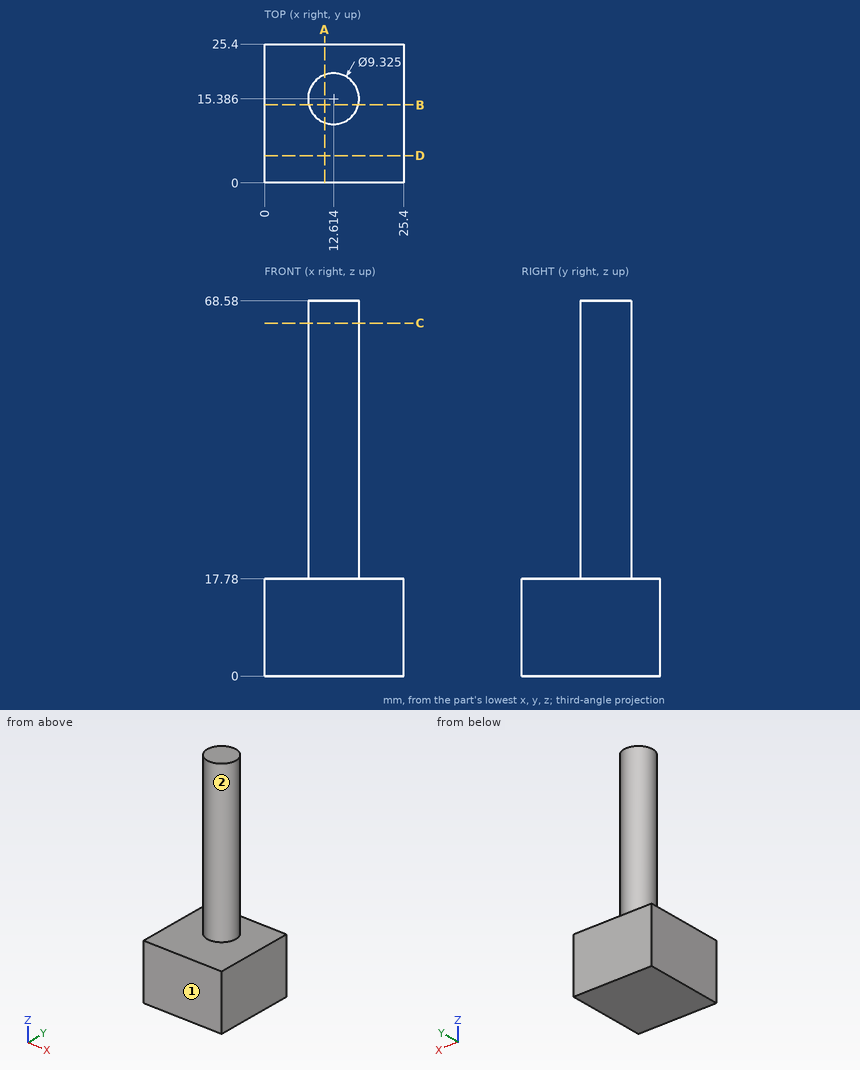
Can you work these out from the drawing? Everything is in mm from the part's minimum corner. A direction names the side the tool comes from. Round coordinates to 2 decimals unless told otherwise and drop trailing zeros. Write each loop counter-clockwise with the first axis right and the second up, starting at its lowest first coordinate (ties: lowest second). Pieces come first, ordered by that corner, then holes. Notation, with made-up numbers: (62, 43.25) - (110, 43.25) arc R24 ccw to (110, 65.25) - close; hole circle Ø3 at (-35.5, 56). An arc over 180 degrees is marked (long way). Write each question's results on one line, items separated by ' | '. Start each with the question number.
1) Suppose I cut it at A-A (x = 11). List the corners of the cut face in (y, z) for me.
2) Suppose I cut it at D-D (y = 5). List the corners of the cut face in (x, z) for me.
3) For pin 1 Ø3 at (y, z) = (19, 19.5) entering from +X; pin 2 Ø4 at (y, z) = (10, 25) entering from -X; pin 3 Ø3 at (y, z) = (16, 61) entering from -X, each with a flat end and sliding along its axis, tell me the tip position at first contact or that it passes through.
4) Suppose I cut it at C-C (z = 64.5). List the corners of the cut face in (x, y) for me (1 decimal).
5) Please list where these lines run through material, in increasing order: line 1 (Z direction, x = 2, y = 19.75); line 2 (X direction, y = 16, z = 61); line 3 (Y direction, x = 9, z = 34.5) (1 decimal).
6) Suppose I cut it at B-B (y = 14.25). List the corners of the cut face in (x, z) for me, and give its area (3 significant figures).
7) Which directions (+Z, -Z, +X, -X, +Y, -Y) give clear straight access to the entire face, cutting with the end or side of a thin tool? Please do the marked faces 1 and 2.
Here are the results:
1) outline: (0, 0) - (25.4, 0) - (25.4, 17.78) - (19.76, 17.78) - (19.76, 68.58) - (11.01, 68.58) - (11.01, 17.78) - (0, 17.78) - close
2) outline: (0, 0) - (25.4, 0) - (25.4, 17.78) - (0, 17.78) - close
3) pin 1: stops at x = 16.77 | pin 2: stops at x = 9.41 | pin 3: stops at x = 7.95
4) outline: circle Ø9.3 at (12.6, 15.4)
5) line 1: z = 0 to 17.78 | line 2: x = 7.99 to 17.24 | line 3: y = 12.4 to 18.3
6) outline: (0, 0) - (25.4, 0) - (25.4, 17.78) - (17.14, 17.78) - (17.14, 68.58) - (8.09, 68.58) - (8.09, 17.78) - (0, 17.78) - close | area: 911 mm2
7) face 1: +Z, -Z, +X, -X, -Y | face 2: +Z
